Check sheet for the modelled part. Datum: model origin and axes. Units: mm. Face numbers are marked on the shaded views. A direction names the side the tool comes from. Round coordinates to 2 decimals unless told otherwise and drop trailing zeros. Write each loop counter-clockwise with the first axis right and the second up, starting at its lowest first coordinate (ties: lowest second). Pieces come first, ordered by that corner, then holes. Notation, with made-up numbers: (-25, 50) -> (-2, 50) arc R19 ccw to (-2, 67) -> close; hole circle Ø6 at (43.5, 49). An arc over 180 degrees is marked (long way). One line per item, written item: value.
from build123d import *

# Parameters (mm, degrees)
BOSS_EXTRUDE1_DEPTH = 100
BOSS_EXTRUDE2_DEPTH = 100
CIRPATTERN1_COUNT   = 6
SKETCH3_W           = 5
SKETCH3_H           = 100
CUT_EXTRUDE1_DEPTH  = 15
CIRPATTERN2_COUNT   = 6
BOSS_EXTRUDE3_DEPTH = 10
SKETCH5_R           = 2.5
CUT_EXTRUDE2_DEPTH  = 200
SKETCH6_R           = 2.5
CUT_EXTRUDE3_DEPTH  = 91.932286341
CIRPATTERN3_COUNT   = 6
BOSS_EXTRUDE4_DEPTH = 100
CIRPATTERN4_COUNT   = 6
BOSS_EXTRUDE5_DEPTH = 10
SKETCH9_R           = 2.5
CUT_EXTRUDE4_DEPTH  = 111


with BuildPart() as part:
    # Sketch1 → Boss-Extrude1 (new body)
    with BuildSketch(Plane(origin=(0, 0, 0), x_dir=(1, 0, 0), z_dir=(0, 1, 0))):
        Polygon((70, 0), (35, 60.621778265), (-35, 60.621778265), (-70, 0), (-35, -60.621778265), (35, -60.621778265), align=None)
    extrude(amount=BOSS_EXTRUDE1_DEPTH)

    # Sketch2 → Boss-Extrude2 (add)
    with BuildSketch(Plane(origin=(0, 100, 0), x_dir=(1, 0, 0), z_dir=(0, 1, 0))):
        Polygon((52.499779997, 73.612286341), (37.500220003, 82.272286341), (24.798707265, 60.272620945), (39.798267258, 51.612620945), align=None)
    boss_extrude2 = extrude(amount=-BOSS_EXTRUDE2_DEPTH)

    # CirPattern1: Boss-Extrude2 ×6 about axis
    cirpattern1_axis = Axis((0, 0, 0), (0, 1, 0))
    for i in range(1, CIRPATTERN1_COUNT):
        add(boss_extrude2.rotate(cirpattern1_axis, i * 360 / CIRPATTERN1_COUNT))

    # Sketch3 → Cut-Extrude1 (cut)
    with BuildSketch(Plane(origin=(90, 0, 0), x_dir=(0, 0, -1), z_dir=(1, 0, 0))):
        with Locations((0, 50)):
            Rectangle(SKETCH3_W, SKETCH3_H)
    cut_extrude1 = extrude(amount=-CUT_EXTRUDE1_DEPTH, mode=Mode.SUBTRACT)

    # CirPattern2: Cut-Extrude1 ×6 about axis
    cirpattern2_axis = Axis((0, 0, 0), (0, 1, 0))
    for i in range(1, CIRPATTERN2_COUNT):
        add(cut_extrude1.rotate(cirpattern2_axis, i * 360 / CIRPATTERN2_COUNT), mode=Mode.SUBTRACT)

    # Sketch4 → Boss-Extrude3 (add)
    with BuildSketch(Plane.XZ):
        Polygon((-52.499779997, 73.612286341), (-37.500220003, 82.272286341), (37.500220003, 82.272286341), (52.499779997, 73.612286341), (90, 8.66), (90, -8.66), (52.499779997, -73.612286341), (37.500220003, -82.272286341), (-37.500220003, -82.272286341), (-52.499779997, -73.612286341), (-90, -8.66), (-90, 8.66), align=None)
        Polygon((50, 0), (25, 43.301270189), (-25, 43.301270189), (-50, 0), (-25, -43.301270189), (25, -43.301270189), align=None, mode=Mode.SUBTRACT)
    extrude(amount=BOSS_EXTRUDE3_DEPTH)

    # Sketch5 → Cut-Extrude2 (cut)
    with BuildSketch(Plane(origin=(0, 100, 0), x_dir=(1, 0, 0), z_dir=(0, 1, 0))):
        Circle(SKETCH5_R)
    extrude(amount=-CUT_EXTRUDE2_DEPTH, mode=Mode.SUBTRACT)

    # Sketch6 → Cut-Extrude3 (cut, through all)
    with BuildSketch(Plane.XY.offset(8.66)):
        with Locations((82.5, 70)):
            Circle(SKETCH6_R)
        with Locations((82.5, 30)):
            Circle(SKETCH6_R)
    cut_extrude3 = extrude(amount=-CUT_EXTRUDE3_DEPTH, mode=Mode.SUBTRACT)

    # CirPattern3: Cut-Extrude3 ×6 about axis
    cirpattern3_axis = Axis((0, -5, 0), (0, 1, 0))
    for i in range(1, CIRPATTERN3_COUNT):
        add(cut_extrude3.rotate(cirpattern3_axis, i * 360 / CIRPATTERN3_COUNT), mode=Mode.SUBTRACT)

    # Sketch7 → Boss-Extrude4 (add)
    with BuildSketch(Plane(origin=(0, 0, 0), x_dir=(1, 0, 0), z_dir=(0, 1, 0))):
        Polygon((-65.000146669, 8.66), (-39.999853331, 51.961778265), (-44.999706662, 60.621778265), (-74.999853331, 8.66), align=None)
    boss_extrude4 = extrude(amount=BOSS_EXTRUDE4_DEPTH)

    # CirPattern4: Boss-Extrude4 ×6 about axis
    cirpattern4_axis = Axis((0, 0, 0), (0, 1, 0))
    for i in range(1, CIRPATTERN4_COUNT):
        add(boss_extrude4.rotate(cirpattern4_axis, i * 360 / CIRPATTERN4_COUNT))

    # Sketch8 → Boss-Extrude5 (add)
    with BuildSketch(Plane.XZ):
        Polygon((50, 0), (25, 43.301270189), (-25, 43.301270189), (-50, 0), (-25, -43.301270189), (25, -43.301270189), align=None)
    extrude(amount=BOSS_EXTRUDE5_DEPTH)

    # Sketch9 → Cut-Extrude4 (cut, through all)
    with BuildSketch(Plane(origin=(0, 100, 0), x_dir=(1, 0, 0), z_dir=(0, 1, 0))):
        Circle(SKETCH9_R)
    extrude(amount=-CUT_EXTRUDE4_DEPTH, mode=Mode.SUBTRACT)


solid = part.part
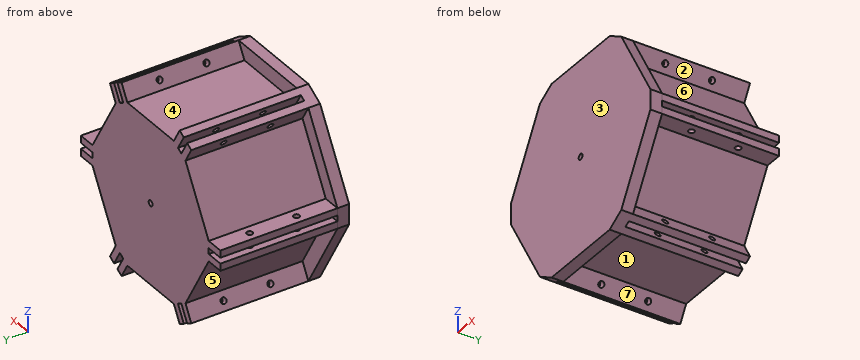
Item 1: Sectioned sample at A-A on y = -3. Enter the section's corners in (x, z), and give its area (3 significant figures).
Answer:
outline: (-90, -8.66) -> (-52.5, -73.61) -> (-37.5, -82.27) -> (37.5, -82.27) -> (52.5, -73.61) -> (90, -8.66) -> (90, 8.66) -> (52.5, 73.61) -> (37.5, 82.27) -> (-37.5, 82.27) -> (-52.5, 73.61) -> (-90, 8.66) -> close; hole circle Ø5 at (0, 0)
area: 23,200 mm^2
Item 2: Sectioned sample at C-C on x = 18.5. Enter the section's corners in (y, z), and give its area (3 significant figures).
Answer:
outline: (-10, -82.27) -> (0, -82.27) -> (0, -69.28) -> (100, -69.28) -> (100, 69.28) -> (0, 69.28) -> (0, 82.27) -> (-10, 82.27) -> close
area: 15,500 mm^2
Item 3: Tool access check on the marked faces 5, 6 and 7. Record the directions out of +Z, -Z, +X, -X, +Y, -Y that give a thin tool (end or side, any length) a straight path to the whole face; none if there is none.
Answer:
face 5: -X, +Y
face 6: +X, +Y
face 7: -Z, +Y
Item 4: Sectioned sample at D-D on z = 50.5. Enter the section's corners in (x, y), and give its area (3 significant figures).
Answer:
outline: (-65.84, -10) -> (65.84, -10) -> (65.84, 0) -> (50.84, 0) -> (50.84, 100) -> (-50.84, 100) -> (-50.84, 0) -> (-65.84, 0) -> close
area: 11,500 mm^2
Item 5: Mould release check, pull along Z, two halves, no side actions. Record for the marked faces 1, 2, 3 and 4: pulls with the +Z half, pulls with the -Z half, needs draft (parallel to the pull), parting line crosses it, or undercut.
Answer:
face 1: pulls with the -Z half
face 2: undercut
face 3: needs draft
face 4: pulls with the +Z half
Item 6: Thickness scan on line 1 (Y direction, x = 82, z = -5); line 2 (Y direction, x = -82.5, z = 7); line 3 (Z direction, x = 82.5, y = 51). Record the ranges inside material, lowest first.
Answer:
line 1: y = -10 to 27.55, 32.45 to 67.55, 72.45 to 100
line 2: y = -10 to 27.5, 32.5 to 67.5, 72.5 to 100
line 3: z = -8.66 to -2.5, 2.5 to 8.66
Item 7: Depth check by flat-ended pin: P1, Ø1, axis at x = 7, y = 20, coming from the +Z side; P2, Ø8, axis at x = -38, y = 18.5, coming from the -Z side; P3, Ø1.5, axis at x = 50.5, y = 74.5, coming from the +Z side; P4, Ø3, axis at x = -82.5, y = 30, coming from the +Z side (3 decimals). Enter the tip coordinate at first touch or a pass-through.
Answer:
P1: stops at z = 69.28
P2: stops at z = -82.27
P3: stops at z = 75.2
P4: passes through
Item 8: Sectioned sample at B-B on z = 0. Enter the section's corners in (x, y), and give its area (4 significant figures).
Answer:
outline: (-90, -10) -> (-2.5, -10) -> (-2.5, 100) -> (-75, 100) -> (-75, 0) -> (-90, 0) -> close; (2.5, -10) -> (90, -10) -> (90, 0) -> (75, 0) -> (75, 100) -> (2.5, 100) -> close
area: 16,250 mm^2
